from build123d import *

# Parameters (mm, degrees)
L_ANGLE_EQUAL_40X40X3_1_DEPTH = 500
CUT_EXTRUDE1_DEPTH            = 504.189825016
CUT_EXTRUDE2_DEPTH            = 504.189825016
SKETCH16_R                    = 2
CUT_EXTRUDE3_DEPTH            = 10


with BuildPart() as part:
    # Sketch11 → L angle (equal) 40X40X3(1) (new body)
    with BuildSketch(Plane(origin=(0, 0, 0), x_dir=(-1, 0, 0), z_dir=(0, 1, 0))):
        with BuildLine():
            Line((0, 40), (0, 0))
            Line((0, 0), (40, 0))
            ThreePointArc((40, 0), (39.121320344, 2.121320344), (37, 3))
            Line((37, 3), (9, 3))
            ThreePointArc((9, 3), (4.757359313, 4.757359313), (3, 9))
            Line((3, 9), (3, 37))
            ThreePointArc((3, 37), (2.121320344, 39.121320344), (0, 40))
        make_face()
    extrude(amount=L_ANGLE_EQUAL_40X40X3_1_DEPTH)

    # Sketch12 → Cut-Extrude1 (cut, through all)
    with BuildSketch(Plane(origin=(0, 0, 0), x_dir=(0, 0, -1), z_dir=(1, 0, 0))):
        Polygon((0, 500), (-40, 500), (-40, 460), align=None)
    extrude(amount=-CUT_EXTRUDE1_DEPTH, mode=Mode.SUBTRACT)

    # Sketch14 → Cut-Extrude2 (cut, through all)
    with BuildSketch(Plane(origin=(0, 0, 0), x_dir=(-1, 0, 0), z_dir=(0, 0, -1))):
        Polygon((40, 40), (0, 0), (40, 0), align=None)
    extrude(amount=-CUT_EXTRUDE2_DEPTH, mode=Mode.SUBTRACT)

    # Sketch16 → Cut-Extrude3 (cut)
    with BuildSketch(Plane(origin=(0, 0, 0), x_dir=(-1, 0, 0), z_dir=(0, 0, -1))):
        with Locations((20, 480)):
            Circle(SKETCH16_R)
        with Locations((20, 20)):
            Circle(SKETCH16_R)
    extrude(amount=-CUT_EXTRUDE3_DEPTH, mode=Mode.SUBTRACT)


solid = part.part
Geometry check sheet. Reference: the model listing, model coordinates, mm. A direction names the side the tool comes from. Round coordinates to 2 decimals unless told otherwise and drop trailing zeros. Loops run counter-clockwise (first coordinate to the right, second up) from the corner with the lowest first, then second, coordinate; pieces in that order, holes last. Notation, with made-up numbers: (-30, 87.5) - (-1, 87.5) arc R26 ccw to (-1, 108.5) - close; hole circle Ø7 at (73, -34.75). An arc over 180 degrees is marked (long way). Answer as CSV lines item,"result".
(1) Material ranges on line 1 along X through (y, z) = (480, 0.6); line 2 along Z through (x, y) = (-31, 333); line 3 along Y through (x, z) = (-20, 1), recorded low to high.
Output values:
line 1,"x = -39.94 to -22, -18 to 0"
line 2,"z = 0 to 3"
line 3,"y = 22 to 478, 482 to 499"
(2) Set-up check for faces 1 (the face through (-23, 250, 3)), 2 (the face through (-2, 2, 14)): record each of +Z, -Z, +X, -X, +Y, -Y from which the full face is reachable in a straight line by a thin tool's end or side.
Output values:
face 1,"+Z, -X, +Y, -Y"
face 2,"+Z, -Z, -X, -Y"
(3) Cross-section at A-A, the plane y = 469. Enter the section's corners in (x, z), and give its area (3 significant figures).
Output values:
outline,"(-40, 0) - (0, 0) - (0, 31) - (-3, 31) - (-3, 9) arc R6 cw to (-9, 3) - (-37, 3) arc R3 ccw to start"
area,"210 mm²"
(4) Cross-section at C-C, the plane x = -26.5. Enter the section's corners in (y, z).
Output values:
outline,"(26.5, 0) - (500, 0) - (497, 3) - (26.5, 3) - close"
(5) Cross-section at B-B, the plane z = 18.5. Enter the section's corners in (x, y).
Output values:
outline,"(-3, 3) - (0, 0) - (0, 481.5) - (-3, 481.5) - close"
(6) Cross-section at D-D, the plane y = 97.5. Enter the section's corners in (x, z).
Output values:
outline,"(-40, 0) - (0, 0) - (0, 40) arc R3 ccw to (-3, 37) - (-3, 9) arc R6 cw to (-9, 3) - (-37, 3) arc R3 ccw to start"
(7) Depth check by flat-ended pin: pin 1 Ø12 at (y, z) = (119.5, 7.5) entering from +X; pin 2 Ø4 at (y, z) = (398, 22.5) entering from -X; pin 3 Ø2 at (y, z) = (88, 6) entering from -X; pin 4 Ø4.5 at (x, y) = (-20, 480) entering from +Z. Enter the tip coordinate at first touch or a pass-through.
Output values:
pin 1,"stops at x = 0"
pin 2,"stops at x = -3"
pin 3,"stops at x = -4.53"
pin 4,"stops at z = 3"
